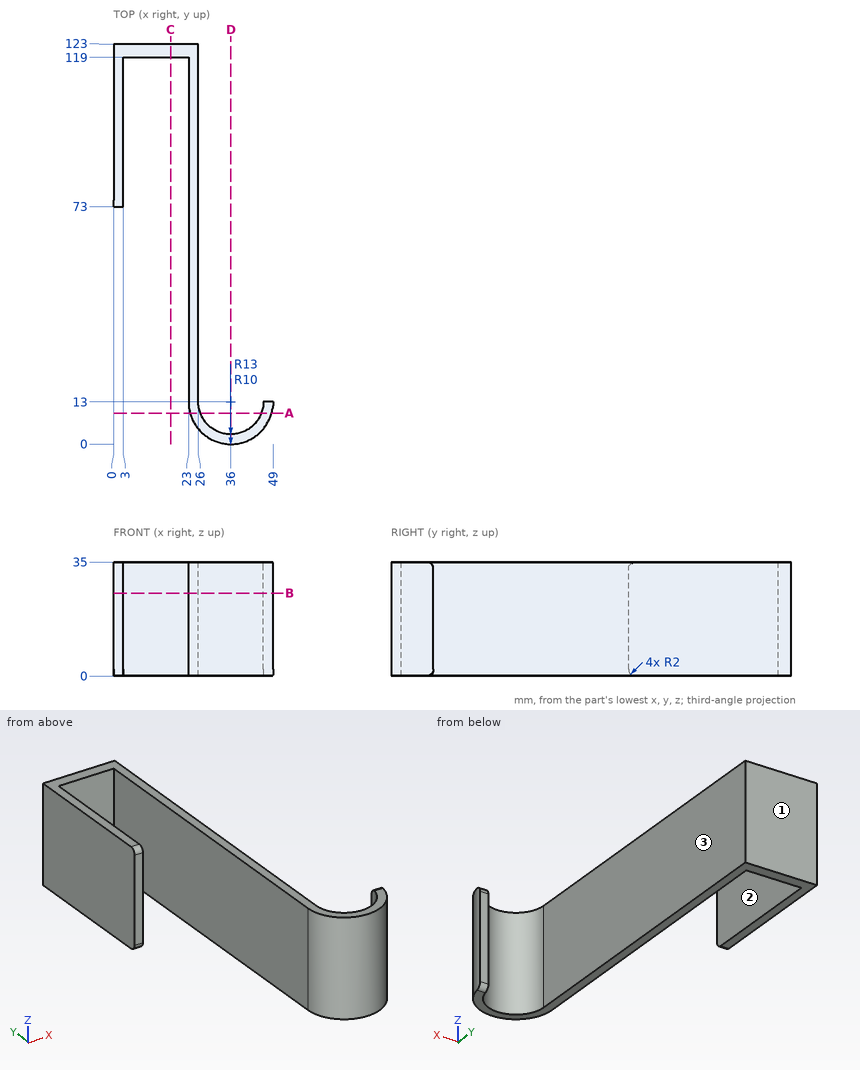
The drawing under review shows one solid part. Ordinate dimensions are in mm from its lowest x, y, z. A direction names the side the tool comes from. Coordinates: 2 decimals unless noted, no trailing zeros. Write each loop counter-clockwise with the first axis right and the second up, starting at its lowest first coordinate (ties: lowest second). Pieces come first, ordered by that corner, then holes. Notation, with made-up numbers: (44.25, 8.25) - (96.25, 8.25) arc R22 cw to (96.25, 16.25) - close; hole circle Ø10 at (26, 72). An arc over 180 degrees is marked (long way). Put each result on its own line as item: value.
1. Wall thickness on probe 1 along X at (y, z) = (110, 31); probe 2 along Y at (x, z) = (36, 2.5); probe 3 along X at (y, z) = (57, 21.5): over which ranges is each line inside the solid? List them lowest first.
Values found:
probe 1: 0 to 3, 23 to 26
probe 2: 0 to 3
probe 3: 23 to 26
2. Add section A-A, the plane y = 9.5. Give the boundary of the cut face in (x, z).
Values found:
outline: (23.48, 0) - (26.63, 0) - (26.63, 35) - (23.48, 35) - close; (45.37, 0) - (48.52, 0) - (48.52, 35) - (45.37, 35) - close
3. Add section C-C, the plane x = 17.5. Give the boundary of the cut face in (y, z), then the cut area to 3 significant figures.
Values found:
outline: (119, 0) - (123, 0) - (123, 35) - (119, 35) - close
area: 140 mm²
4. Machinability: for the marked faces 1, 2 and 3, which of the approach directions +Z, -Z, +X, -X, +Y, -Y give a long, thin tool a straight path to every point of the face, cutting with its end or side? Answer none if there is none.
Values found:
face 1: +Z, -Z, +X, -X, +Y
face 2: +Z, -Z, -Y
face 3: +Z, -Z, +X, +Y
5. For pin 1 (4 mm diameter, centred on x = 28.5, z = 22.5, fed in from -Y); pin 2 (6 mm diameter, centred on x = 11.5, z = 19.5, fed in from -Y); pin 3 (8 mm diameter, centred on y = 104, z = 30.5, fed in from +X); pin 4 (5 mm diameter, centred on y = 89.5, z = 29.5, fed in from -X), all flat-tipped, find the tip position at first contact; note any pin that passes through.
Values found:
pin 1: y = 1.22
pin 2: y = 119
pin 3: x = 26
pin 4: x = 0
6. Add section B-B, the plane z = 25.5. Give the boundary of the cut face in (x, y).
Values found:
outline: (0, 73) - (3, 73) - (3, 119) - (23, 119) - (23, 13) arc R13 ccw to (49, 13) - (46, 13) arc R10 cw to (26, 13) - (26, 123) - (0, 123) - close
7. Add section D-D, the plane x = 36. Give the boundary of the cut face in (y, z), then the cut area to 3 significant figures.
Values found:
outline: (0, 0) - (3, 0) - (3, 35) - (0, 35) - close
area: 105 mm²
